The listing builds one solid part. Answer for the finished solid, in the listing's coordinates (mm). A direction names the side the tool comes from. Coordinates: 2 decimals unless noted, no trailing zeros. Put each result on its own line as item: value. Start each with the question number.
```python
from build123d import *

# Parameters (mm, degrees)
F0_W      = 75
F0_H      = 63
F1_DEPTH  = 7
F3_DEPTH  = 25
F5_DEPTH  = 25
F7_W      = 52
F7_H      = 11
F8_DEPTH  = 2.5
F10_DEPTH = 80
F12_DEPTH = 25


with BuildPart() as f1:
    # F0 (on Top) → F1 (new body)
    with BuildSketch(Plane.XY):
        Rectangle(F0_W, F0_H)
    extrude(amount=F1_DEPTH)

    # F2 (on face) → F3 (cut)
    with BuildSketch(Plane.XY.offset(7)):
        Polygon((27, 18.5), (-27, 18.5), (-27, 7.5), (-30.75, 7.5), (-30.75, -11.5), (-12.75, -11.5), (-10.75, -9), (10.75, -9), (12.75, -11.5), (30.75, -11.5), (30.75, 7.5), (27, 7.5), align=None)
    extrude(amount=-F3_DEPTH, mode=Mode.SUBTRACT)

    # F4 (on face) → F5 (cut)
    with BuildSketch(Plane.XY.offset(7)):
        with BuildLine():
            Line((-26, -18), (-26, -20.5))
            Line((-26, -20.5), (26, -20.5))
            Line((26, -20.5), (26, -18))
            add(Edge.make_bspline(
                [(-26, -18), (-11, -17), (0, -17), (11, -17), (26, -18)],
                knots=[0, 0, 0, 0, 0.5, 1, 1, 1, 1], degree=3))
        make_face()
    extrude(amount=-F5_DEPTH, mode=Mode.SUBTRACT)

    # F7 (on face) → F8 (cut)
    with BuildSketch(Plane.XY.offset(7)):
        with Locations((0, -26)):
            Rectangle(F7_W, F7_H)
    extrude(amount=-F8_DEPTH, mode=Mode.SUBTRACT)

    # F9 (on face) → F10 (cut)
    with BuildSketch(Plane.YZ.offset(37.5)):
        with BuildLine():
            Line((-31.5, 11.1092058942), (-31.5, 7))
            Line((-31.5, 7), (13.5, 7))
            add(Edge.make_bspline(
                [(31.5, 2), (27.9249660671, 4.0678475052), (24.5989065318, 5.4442587825), (16.5555038096, 6.4860110295), (13.5, 7)],
                knots=[0, 0, 0, 0, 0.4750633648, 1, 1, 1, 1], degree=3))
            Line((31.5, 2), (31.5, 11.1092058942))
            Line((31.5, 11.1092058942), (-31.5, 11.1092058942))
        make_face()
    extrude(amount=-F10_DEPTH, mode=Mode.SUBTRACT)

    # F11 (on Top) → F12 (cut)
    with BuildSketch(Plane.XY):
        with BuildLine():
            add(Edge.make_bspline(
                [(-31, 31.5), (-35.5, 21.5), (-39.5000541268, 0.1581786089), (-35.5, -21.5), (-34, -31.5)],
                knots=[0, 0, 0, 0, 0.5018392613, 1, 1, 1, 1], degree=3))
            Line((-31, 31.5), (-43.3181733368, 37.5741338942))
            Line((-43.3181733368, 37.5741338942), (-41.833250428, -36.0357076911))
            Line((-41.833250428, -36.0357076911), (-34, -31.5))
        make_face()
        with BuildLine():
            Line((39.6972207541, 40.7548360527), (31.0000020678, 31.5))
            add(Edge.make_bspline(
                [(31.0000020678, 31.5), (35.5, 21.5), (39.5000541267, 0.1581784693), (35.5, -21.5), (34, -31.5)],
                knots=[0, 0, 0, 0, 0.5018392596, 1, 1, 1, 1], degree=3))
            Line((34, -31.5), (45.6182770431, -33.850427717))
            Line((45.6182770431, -33.850427717), (39.6972207541, 40.7548360527))
        make_face()
    extrude(amount=F12_DEPTH, mode=Mode.SUBTRACT)

    # F13: F1 across plane


with BuildPart() as f1_1:
    add(f1.part)
    add(f1.part.mirror(Plane.XY))


solid = f1_1.part
```
(1) For a pull along X with two mould halves and no side action, classify faces 1 (the flat face through (29, 7.5, 0)), 2 (the flat face through (0, -31.5, 0)) as released by +X, released by -X, zero draft, split by the parting line, or undercut.
(2) A tool of negligible diameter and unlimited length cuts with its end or side. For faces 3 (the flat face through (-29, 7.5, 0)), 4 (the flat face through (26, -20, 0)), 5 (the flat face through (0, -26, -4.5)), 6 (the flat face through (0, -11, -7)), 7 (the flat face through (0, -26, 4.5)), from which of +Z, -Z, +X, -X, +Y, -Y can it reach the whole face along a straight path? Write none if from no direction.
(3) Find the intervals of material crossed by L1, parallel to Y at x = 24, z = -1.5; L2, parallel to Y at x = -18.5, z = 0.25; L3, parallel to Y at x = 28.5, z = -1.5, in increasing order.
(4) Each of these flat-tipped pins is pushed along its axis until it touches: P1, Ø5.5, axis at y = 10.5, z = 1, coming from the -X side; P2, Ø7, axis at y = -24.5, z = -3, coming from the +X side; P3, Ø1.5, axis at x = -18.5, y = 17, coming from the +Z side; P4, Ø1, axis at y = 3, z = 2, coming from the -X side. Where does it stop, or does it pass through?
(5) The part is cut by section A-A on x = 21. Count the separate pieces of the cut face and the enclosed holes in it, plus the area to 3 significant figures.
Worked out:
1. face 1: undercut
1. face 2: zero draft
2. face 3: +Z, -Z
2. face 4: none
2. face 5: -Z, -Y
2. face 6: -Z, +X, -X, +Y, -Y
2. face 7: +Z, -Y
3. L1: -31.5 to -20.5, -17.87 to -11.5, 18.5 to 31.5
3. L2: -31.5 to -20.5, -17.54 to -11.5, 18.5 to 31.5
3. L3: -31.5 to -11.5, 7.5 to 31.5
4. P1: x = -37.15
4. P2: x = 35.61
4. P3: through
4. P4: x = -37.47
5. separate pieces: 3
5. enclosed holes: 0
5. area: 307 mm2
